```python
from build123d import *

# Parameters (mm, degrees)
SKETCH1_R           = 16
BOSS_EXTRUDE1_DEPTH = 6.35
FILLET1_R           = 10
SKETCH2_W           = 48
SKETCH2_H           = 20
BOSS_EXTRUDE2_DEPTH = 6.35
SKETCH4_W           = 6.35
SKETCH4_H           = 33.563954303
BOSS_EXTRUDE3_DEPTH = 6
SKETCH5_R           = 1.976318005
CUT_EXTRUDE1_DEPTH  = 85.265533897
SKETCH6_R           = 0.818763353
CUT_EXTRUDE2_DEPTH  = 4
CUT_EXTRUDE3_DEPTH  = 85.265533897
FILLET2_R           = 10


with BuildPart() as part:
    # Sketch1 → Boss-Extrude1 (new body)
    with BuildSketch(Plane.XY):
        with BuildLine():
            Line((15.771494463, -0.425728707), (39.940720481, -0.425728707))
            Line((39.940720481, -0.425728707), (39.940720481, 14.222654346))
            ThreePointArc((39.940720481, 14.222654346), (46.645253692, 42.541279088), (17.982311374, 47.574271293))
            Line((17.982311374, 47.574271293), (-8.059279519, 47.574271293))
            Line((-8.059279519, 47.574271293), (-8.059279519, 27.711945938))
            ThreePointArc((-8.059279519, 27.711945938), (-17.321126946, -4.292626776), (15.771494463, -0.425728707))
        make_face()
        with Locations((-2.059279519, 8.63316191)):
            Circle(SKETCH1_R, mode=Mode.SUBTRACT)
        with Locations((29.940720481, 31.543162422)):
            Circle(SKETCH1_R, mode=Mode.SUBTRACT)
    extrude(amount=BOSS_EXTRUDE1_DEPTH)

    # Fillet1
    fillet1_edges = [part.edges().sort_by_distance(p)[0] for p in [
        (17.982311374, 47.574271293, 3.175),
        (39.940720481, 14.222654346, 3.175),
        (15.771494463, -0.425728707, 3.175),
        (-8.059279519, 27.711945938, 3.175),
    ]]
    fillet(fillet1_edges, radius=FILLET1_R)

    # Sketch2 → Boss-Extrude2 (add)
    with BuildSketch(Plane(origin=(0, 0, 0), x_dir=(-1, 0, 0), z_dir=(0, 0, -1))):
        with Locations((-15.940720481, 57.574271293)):
            Rectangle(SKETCH2_W, SKETCH2_H)
        with BuildLine():
            Line((-39.940720481, -0.425728707), (-39.940720481, -20.425728707))
            Line((-39.940720481, -20.425728707), (8.059279519, -20.425728707))
            Line((8.059279519, -20.425728707), (8.059279519, -6.199235065))
            ThreePointArc((8.059279519, -6.199235065), (-2.550706673, -6.68832716), (-11.129219288, -0.425728707))
            Line((-11.129219288, -0.425728707), (-39.940720481, -0.425728707))
        make_face()
    extrude(amount=-BOSS_EXTRUDE2_DEPTH)

    # Sketch4 → Boss-Extrude3 (add)
    with BuildSketch(Plane.ZY.offset(8.059279519)):
        with Locations((3.175, 50.792294142)):
            Rectangle(SKETCH4_W, SKETCH4_H)
    extrude(amount=BOSS_EXTRUDE3_DEPTH)

    # Sketch5 → Cut-Extrude1 (cut, through all)
    with BuildSketch(Plane.XY.offset(6.35)):
        with Locations((31.940720481, 63.574271293)):
            Circle(SKETCH5_R)
        with Locations((-0.059279519, 63.574271293)):
            Circle(SKETCH5_R)
        with Locations((23.940720481, 7.574271293)):
            Circle(SKETCH5_R)
        with Locations((7.455439106, 32.059552667)):
            Circle(SKETCH5_R)
    extrude(amount=-CUT_EXTRUDE1_DEPTH, mode=Mode.SUBTRACT)

    # Sketch6 → Cut-Extrude2 (cut)
    with BuildSketch(Plane.ZY.offset(14.059279519)):
        with Locations(Location((2.747841942, 62.56121214, 0), (0, 0, 270))):
            Circle(SKETCH6_R)
        with Locations(Location((2.756756589, 51.313832117, 0), (0, 0, 270))):
            Circle(SKETCH6_R)
        with Locations(Location((2.756756589, 40.313832117, 0), (0, 0, 270))):
            Circle(SKETCH6_R)
    extrude(amount=-CUT_EXTRUDE2_DEPTH, mode=Mode.SUBTRACT)

    # Sketch7 → Cut-Extrude3 (cut, through all)
    with BuildSketch(Plane(origin=(0, 0, 0), x_dir=(-1, 0, 0), z_dir=(0, 0, -1))):
        Polygon((-40.812011189, 13.264965551), (-6.140614995, -23.185471789), (-44.163616568, -23.185471789), (-44.163616568, 13.264965551), align=None)
    extrude(amount=-CUT_EXTRUDE3_DEPTH, mode=Mode.SUBTRACT)

    # Fillet2
    # the kernel refuses this fillet: 10 mm, written as the material it takes off along each edge
    with BuildSketch(Plane(origin=(-8.059279519, -20.425728707, -25), x_dir=(1, 0, 0), z_dir=(0, 0, 1))) as fillet2_piece_1_section:
        with BuildLine():
            CenterArc((FILLET2_R, FILLET2_R), FILLET2_R, 180, 90)
            Line((0, FILLET2_R), (0, 0))
            Line((0, 0), (FILLET2_R, 0))
        make_face()
    fillet2_piece_1 = extrude(amount=56.35, mode=Mode.PRIVATE)
    fillet2_piece_1 = fillet2_piece_1 - Plane(origin=(-2.059279519, 8.63316191, 3.175), x_dir=(-0.30000000000000054, 0.9539392014169455, 0), z_dir=(0, 0, -1)) * Cylinder(20, 153, mode=Mode.PRIVATE)
    add(fillet2_piece_1, mode=Mode.SUBTRACT)
    with BuildSketch(Plane(origin=(8.765662944, -20.425728707, -10.72351028), x_dir=(0.6892036325040336, 0.7245677007314395, 0), z_dir=(0, 0, 1))) as fillet2_piece_2:
        with BuildLine():
            CenterArc((FILLET2_R * 0.428940411203, FILLET2_R), FILLET2_R, 223.567102496, 46.432897504)
            Line((-FILLET2_R * 0.295627289529, FILLET2_R * 0.310796367496), (0, 0))
            Line((0, 0), (FILLET2_R * 0.428940411203, 0))
        make_face()
    extrude(amount=27.79702056, mode=Mode.SUBTRACT)


solid = part.part
```
For this review, take the finished solid that the model builds, in its own axes (mm). A direction names the side the tool comes from. Round coordinates to 2 decimals unless told otherwise and drop trailing zeros. Write each loop counter-clockwise with the first axis right and the second up, starting at its lowest first coordinate (ties: lowest second). Pieces come first, ordered by that corner, then holes. Notation, with made-up numbers: M 52,-28 L 106,-28 A17 ccw 106,-17 Z; hole C 48.25,45 d6. An arc over 180 degrees is marked long. One line per item, written item: value. Start each with the question number.
(1) Insertion check: pin 1 (1.3 mm diameter, centred on y = 51.5, z = 3, fed in from -X); pin 2 (1 mm diameter, centred on y = 51.31, z = 2.76, fed in from -X); pin 3 (1 mm diameter, centred on y = 52, z = 1, fed in from +X); pin 4 (3.5 mm diameter, centred on x = 31.94, y = 63.57, fed in from +Z). Each pin has a flat end and moves straight along its axis. Give the tip position at first contact, or say it passes through.
(2) We need section C-C (x = 24.5). Give the boundary of the cut face in (y, z).
(3) The part is to be moulded in two halves that separate along X. For faces 4 (the cylindrical face through (17.24, 21.81, 3.13)), 5 (the flat face through (26.471, -1.812, 3.131)), 6 (the flat face through (-14.059, 51, 4)), say which applies: released by +X, released by -X, zero draft, split by the parting line, or undercut.
(4) Wall thickness on line 1 (Y direction, x = -11.5, z = 2.25); line 2 (Y direction, x = 6, z = 4); line 3 (X direction, y = 30.5, z = 5.25): over which ranges is each line inside the solid? List them lowest first.
(5) We need section A-A (x = 37). Give the boundary of the cut face in (y, z), and give its area (3 significant figures).
(6) Machinability: for faces 1 (the cylindrical face through (8.366, -19.638, 3.131)), 2 (the flat face through (39.941, 58, 3)), 3 (the cylindrical face through (-9.338, 29.118, 3.219)), which of the approach directions +Z, -Z, +X, -X, +Y, -Y give a long, thin tool a straight path to every point of the face, cutting with its end or side? Answer none if there is none.
(7) We need section B-B (y = 28.5). Give the boundary of the cut face in (x, z).
(8) We need section D-D (z = 5.25). Give the boundary of the cut face in (x, y).
Result:
1. pin 1: x = -14.06
1. pin 2: x = -10.06
1. pin 3: x = 39.94
1. pin 4: through
2. outline: M -3.88,0 L 5.68,0 L 5.68,6.35 L -3.88,6.35 Z; M 9.47,0 L 16.5,0 L 16.5,6.35 L 9.47,6.35 Z; M 46.59,0 L 67.57,0 L 67.57,6.35 L 46.59,6.35 Z
3. face 4: undercut
3. face 5: released by +X
3. face 6: released by -X
4. line 1: -9 to -4.28, 21.55 to 26.46, 34.01 to 39.67, 40.96 to 50.67, 51.96 to 61.91, 63.21 to 67.57
4. line 2: -20.31 to -5.19, 22.46 to 30.72, 33.4 to 67.57
4. line 3: -8.7 to 6.24, 8.67 to 13.97, 45.91 to 49.91
5. outline: M 9.26,0 L 17.18,0 L 17.18,6.35 L 9.26,6.35 Z; M 45.9,0 L 67.57,0 L 67.57,6.35 L 45.9,6.35 Z
5. area: 188 mm²
6. face 1: +Z, -Z, +X, -Y
6. face 2: +Z, -Z, +X, +Y
6. face 3: +Z, -Z, -X
7. outline: M -9.71,0 L 14.23,0 L 14.23,6.35 L -9.71,6.35 Z; M 45.65,0 L 49.71,0 L 49.71,6.35 L 45.65,6.35 Z
8. outline: M -14.06,34.01 L -8.06,34.01 A10 cw -12.73,25.55 A20 ccw -8.06,-10.45 A10 ccw 1.94,-20.43 L 4.48,-20.43 A10 ccw 11.72,-17.32 L 40.81,13.26 A10 cw 43.27,16.64 A20 ccw 39.94,48.86 L 39.94,67.57 L -14.06,67.57 Z; hole C -2.06,8.63 d32; hole C -0.06,63.57 d3.95; hole C 7.46,32.06 d3.95; hole C 29.94,31.54 d32; hole C 23.94,7.57 d3.95; hole C 31.94,63.57 d3.95
